Can you work these out from the model? Positions are in its coordinate system, mm. A direction names the side the tool comes from. Round coordinates to 2 decimals unless told otherwise and drop trailing zeros. Loops run counter-clockwise (first coordinate to the right, second up) from the corner with the lowest first, then second, coordinate; pieces in that order, holes last. Notation, with made-up numbers: (6.5, -37.75) - (32.5, -37.75) arc R21 cw to (32.5, -1.75) - close; hole circle Ø5 at (55, 33). An arc over 180 degrees is marked (long way). Answer as CSV lines item,"result".
```python
from build123d import *

# Parameters (mm, degrees)
SKETCH_1_W          = 99.5
SKETCH_1_H          = 15
EXTRUDE_1_DEPTH     = 15
SKETCH_2_R          = 2.2
CUT_EXTRUDE_1_DEPTH = 55
CUT_EXTRUDE_2_DEPTH = 48
FILLET_1_R          = 2
CUT_EXTRUDE_3_DEPTH = 31


with BuildPart() as part:
    # 草图1 → 凸台-拉伸1 (new body)
    with BuildSketch(Plane(origin=(0, 0, 0), x_dir=(0, 0, -1), z_dir=(1, 0, 0))):
        with Locations((49.75, -7.5)):
            Rectangle(SKETCH_1_W, SKETCH_1_H)
    extrude(amount=EXTRUDE_1_DEPTH)

    # 草图2 → 切除-拉伸1 (cut)
    with BuildSketch(Plane(origin=(15, 0, 0), x_dir=(0, 0, -1), z_dir=(1, 0, 0))):
        with Locations((49.75, -7.5)):
            Circle(SKETCH_2_R)
        with Locations((11.25, -7.5)):
            Circle(SKETCH_2_R)
        with Locations((88.25, -7.5)):
            Circle(SKETCH_2_R)
    extrude(amount=-CUT_EXTRUDE_1_DEPTH, mode=Mode.SUBTRACT)

    # 草图3 → 切除-拉伸2 (cut)
    with BuildSketch(Plane(origin=(15, 0, 0), x_dir=(0, 0, -1), z_dir=(1, 0, 0))):
        with BuildLine():
            Line((21.25, -2.5), (39.75, -2.5))
            ThreePointArc((39.75, -2.5), (44.75, -7.5), (39.75, -12.5))
            Line((39.75, -12.5), (21.25, -12.5))
            ThreePointArc((21.25, -12.5), (16.25, -7.5), (21.25, -2.5))
        make_face()
        with BuildLine():
            Line((59.75, -2.5), (78.25, -2.5))
            ThreePointArc((78.25, -2.5), (83.25, -7.5), (78.25, -12.5))
            Line((78.25, -12.5), (59.75, -12.5))
            ThreePointArc((59.75, -12.5), (54.75, -7.5), (59.75, -2.5))
        make_face()
    extrude(amount=-CUT_EXTRUDE_2_DEPTH, mode=Mode.SUBTRACT)

    # 圆角1
    fillet_1_edges = [part.edges().sort_by_distance(p)[0] for p in [
        (7.5, 0, 0),
        (7.5, 0, -99.5),
        (7.5, -15, -99.5),
        (7.5, -15, 0),
    ]]
    fillet(fillet_1_edges, radius=FILLET_1_R)

    # 草图4 → 切除-拉伸3 (cut)
    with BuildSketch(Plane(origin=(0, 0, 0), x_dir=(1, 0, 0), z_dir=(0, 1, 0))):
        with BuildLine():
            ThreePointArc((7.25, 22.75), (6.590990258, 24.340990258), (5, 25))
            Line((5, 25), (5, 20.5))
            ThreePointArc((5, 20.5), (6.590990258, 21.159009742), (7.25, 22.75))
        make_face()
        with BuildLine():
            Line((5, 20.5), (5, 25))
            ThreePointArc((5, 25), (2.75, 22.75), (5, 20.5))
        make_face()
        with BuildLine():
            ThreePointArc((7.25, 76.75), (6.590990258, 78.340990258), (5, 79))
            Line((5, 79), (5, 74.5))
            ThreePointArc((5, 74.5), (6.590990258, 75.159009742), (7.25, 76.75))
        make_face()
        with BuildLine():
            Line((5, 74.5), (5, 79))
            ThreePointArc((5, 79), (2.75, 76.75), (5, 74.5))
        make_face()
    extrude(amount=-CUT_EXTRUDE_3_DEPTH, mode=Mode.SUBTRACT)


solid = part.part
```
Q1. Imagine slicing it at D-D (y = -14). Write out the boundary of the cut face in (x, z), then the cut area to 3 significant figures.
Checks:
outline,"(0, -99.23) - (15, -99.23) - (15, -0.27) - (0, -0.27) - close; hole circle Ø4.5 at (5, -76.75); hole circle Ø4.5 at (5, -22.75)"
area,"1,450 mm²"
Q2. On a 3-axis mill with a long thin cutter (end or side, diameter ignored), from which of +Z, -Z, +X, -X, +Y, -Y can I reach the whole of each face in a straight line? I mean faces 4 (the cylindrical face through (7.6, -0.57, -98.9)), 5 (the flat face through (8, -2.5, -30)). Say none if no direction works.
Checks:
face 4,"-Z, +X, -X, +Y"
face 5,"+X, -X"
Q3. I'm going to push flat-ended pins straight in: pin 1 Ø4 at (y, z) = (-7.5, -49.75) entering from +X; pin 2 Ø7 at (y, z) = (-7.5, -88.25) entering from +X. Where does each tip first touch, or does it pass through?
Checks:
pin 1,"through"
pin 2,"x = 15"
Q4. We'd pull the mould along Y, two halves only. Please class faces 1 (the flat face through (8, -12.5, -69)), 2 (the flat face through (7, 0, -49)), 3 (the cylindrical face through (7.6, -14.43, -98.9)): pulls with the +Y half, pulls with the -Y half, needs draft (parallel to the pull), parting line crosses it, or undercut.
Checks:
face 1,"undercut"
face 2,"pulls with the +Y half"
face 3,"pulls with the -Y half"
Q5. Imagine slicing it at A-A (z = -64). Write out the boundary of the cut face in (x, y).
Checks:
outline,"(0, -15) - (15, -15) - (15, -12.5) - (0, -12.5) - close; (0, -2.5) - (15, -2.5) - (15, 0) - (0, 0) - close"
Q6. If I drill on line 1 along Y through (x, z) = (6.75, -49.75); line 2 along Z through (x, y) = (14.25, -6); line 3 along Z through (x, y) = (1.25, -4.25), over which ranges is the centre line in solid material (lowest first)? Write a range as [from, to].
Checks:
line 1,"[-15, -9.7], [-5.3, 0]"
line 2,"[-99.5, -89.86], [-86.64, -83.02], [-54.98, -51.36], [-48.14, -44.52], [-16.48, -12.86], [-9.64, 0]"
line 3,"[-99.5, -82.05], [-55.95, -43.55], [-17.45, 0]"
Q7. Imagine slicing it at B-B (x = 10.75). Write out the boundary of the cut face in (y, z).
Checks:
outline,"(-15, -97.5) arc R2 ccw to (-13, -99.5) - (-2, -99.5) arc R2 ccw to (0, -97.5) - (0, -2) arc R2 ccw to (-2, 0) - (-13, 0) arc R2 ccw to (-15, -2) - close; hole (-12.5, -78.25) arc R5 ccw to (-2.5, -78.25) - (-2.5, -59.75) arc R5 ccw to (-12.5, -59.75) - close; hole (-12.5, -39.75) arc R5 ccw to (-2.5, -39.75) - (-2.5, -21.25) arc R5 ccw to (-12.5, -21.25) - close; hole circle Ø4.4 at (-7.5, -88.25); hole circle Ø4.4 at (-7.5, -49.75); hole circle Ø4.4 at (-7.5, -11.25)"
Q8. Imagine slicing it at C-C (y = -7.5). Write out the boundary of the cut face in (x, z).
Checks:
outline,"(0, -99.5) - (15, -99.5) - (15, -90.45) - (0, -90.45) - close; (0, -86.05) - (15, -86.05) - (15, -83.25) - (0, -83.25) - close; (0, -54.75) - (15, -54.75) - (15, -51.95) - (0, -51.95) - close; (0, -47.55) - (15, -47.55) - (15, -44.75) - (0, -44.75) - close; (0, -16.25) - (15, -16.25) - (15, -13.45) - (0, -13.45) - close; (0, -9.05) - (15, -9.05) - (15, 0) - (0, 0) - close"
